from build123d import *

# Parameters (mm, degrees)
BOSS_EXTRUDE1_DEPTH = 30
SKETCH2_W           = 2.5
SKETCH2_H           = 5
CUT_EXTRUDE1_DEPTH  = 5
SKETCH3_R           = 8.1
CUT_EXTRUDE2_DEPTH  = 71
BOSS_EXTRUDE5_DEPTH = 4
CUT_EXTRUDE3_DEPTH  = 2
FILLET1_R           = 2


with BuildPart() as part:
    # Sketch1 → Boss-Extrude1 (new body)
    with BuildSketch(Plane(origin=(0, 0, 0), x_dir=(1, 0, 0), z_dir=(0, 1, 0))):
        with BuildLine():
            Line((8, -65), (8, 0))
            Line((8, 0), (58, 0))
            Line((58, 0), (58, -6.5))
            Line((58, -6.5), (55, -6.5))
            ThreePointArc((55, -6.5), (54.292893219, -6.792893219), (54, -7.5))
            Line((54, -7.5), (54, -9))
            ThreePointArc((54, -9), (54.292893219, -9.707106781), (55, -10))
            Line((55, -10), (60, -10))
            ThreePointArc((60, -10), (61.414213562, -9.414213562), (62, -8))
            Line((62, -8), (62, 0))
            Line((62, 0), (116, 0))
            Line((116, 0), (116, 5))
            Line((116, 5), (0, 5))
            Line((0, 5), (0, -10))
            Line((0, -10), (5, -10))
            Line((5, -10), (5, -57.5))
            Line((5, -57.5), (0, -57.5))
            Line((0, -57.5), (0, -63))
            ThreePointArc((0, -63), (0.585786438, -64.414213562), (2, -65))
            Line((2, -65), (8, -65))
        make_face()
    extrude(amount=BOSS_EXTRUDE1_DEPTH)

    # Sketch2 → Cut-Extrude1 (cut)
    with BuildSketch(Plane.ZY):
        with Locations((8.75, 15)):
            Rectangle(SKETCH2_W, SKETCH2_H)
        with Locations((58.75, 15)):
            Rectangle(SKETCH2_W, SKETCH2_H)
    extrude(amount=-CUT_EXTRUDE1_DEPTH, mode=Mode.SUBTRACT)

    # Sketch3 → Cut-Extrude2 (cut, through all)
    with BuildSketch(Plane(origin=(0, 0, -5), x_dir=(-1, 0, 0), z_dir=(0, 0, -1))):
        with Locations((-103, 12)):
            Circle(SKETCH3_R)
        with Locations((-75.8, 12)):
            Circle(SKETCH3_R)
    extrude(amount=-CUT_EXTRUDE2_DEPTH, mode=Mode.SUBTRACT)

    # Sketch8 → Boss-Extrude5 (add)
    with BuildSketch(Plane(origin=(116, 0, 0), x_dir=(0, 0, -1), z_dir=(1, 0, 0))):
        with BuildLine():
            Line((-8, 36), (-9.664100589, 33.503849117))
            ThreePointArc((-9.664100589, 33.503849117), (-9.914184053, 32.974017022), (-10, 32.394448725))
            Line((-10, 32.394448725), (-10, 30.32455532))
            ThreePointArc((-10, 30.32455532), (-9.974174915, 30.004190834), (-9.897366596, 29.692099788))
            Line((-9.897366596, 29.692099788), (0, 0))
            Line((0, 0), (0, 30))
            Line((0, 30), (-6, 30))
            Line((-6, 30), (-6, 36))
            Line((-6, 36), (-8, 36))
        make_face()
        with BuildLine():
            Line((5, 30), (5, 34))
            ThreePointArc((5, 34), (4.414213562, 35.414213562), (3, 36))
            Line((3, 36), (0, 36))
            Line((0, 36), (0, 30))
            Line((0, 30), (5, 30))
        make_face()
    extrude(amount=-BOSS_EXTRUDE5_DEPTH)

    # Sketch10 → Cut-Extrude3 (cut)
    with BuildSketch(Plane(origin=(0, 0, -5), x_dir=(-1, 0, 0), z_dir=(0, 0, -1))):
        Polygon((-112, 30), (-113, 25), (-113, 1.5), (-65.8, 1.5), (-65.8, 26), (0, 26), (0, 30), align=None)
        with BuildLine():
            ThreePointArc((-93, 16), (-92.414213562, 17.414213562), (-91, 18))
            Line((-91, 18), (-87.8, 18))
            ThreePointArc((-87.8, 18), (-86.385786438, 17.414213562), (-85.8, 16))
            Line((-85.8, 16), (-85.8, 10))
            ThreePointArc((-85.8, 10), (-86.385786438, 8.585786438), (-87.8, 8))
            Line((-87.8, 8), (-91, 8))
            ThreePointArc((-91, 8), (-92.414213562, 8.585786438), (-93, 10))
            Line((-93, 10), (-93, 16))
        make_face(mode=Mode.SUBTRACT)
    extrude(amount=-CUT_EXTRUDE3_DEPTH, mode=Mode.SUBTRACT)

    # Fillet1
    fillet1_edges = [part.edges().sort_by_distance(p)[0] for p in [
        (0, 13, -5),
        (0, 28, -3),
    ]]
    fillet(fillet1_edges, radius=FILLET1_R)


solid = part.part
The listing builds one solid part. Answer for the finished solid, in the listing's coordinates (mm). A direction names the side the tool comes from. Coordinates: 2 decimals unless noted, no trailing zeros. Write each loop counter-clockwise with the first axis right and the second up, starting at its lowest first coordinate (ties: lowest second). Pieces come first, ordered by that corner, then holes. Notation, with made-up numbers: M 70.25,-11 L 79.25,-11 A25 cw 79.25,1 Z; hole C 41.5,64 d9. An arc over 180 degrees is marked long. Put each result on its own line as item: value. Start each with the question number.
1. A cutting plane is placed at C-C on y = 28. Write down the section's boundary in (x, z), then the cut area to 3 significant figures.
2. Flat-ended cylindrical pins translate along their axes: P1, Ø10, axis at y = 22.5, z = 58, coming from the -X side; P2, Ø8, axis at x = 29, y = 29, coming from the +Z side; P3, Ø13, axis at x = 103, y = 12, coming from the -Z side; P4, Ø10, axis at y = 13.5, z = 11.5, coming from the +X side. Find the tip coordinate at first contact, or state that the pin passes through.
3. Which of the six approach directions +Z, -Z, +X, -X, +Y, -Y give full straight-line access (tool end or side, diameter ignored) to faces 1 (the flat face through (31, 30, -2)), 2 (the flat face through (2, 12.5, 59)), 3 (the flat face through (3, 24, 57.5)), 4 (the flat face through (62, 15, 4)), 5 (the flat face through (114, 33, 6))?
4. A cutting plane is placed at A-A on z = 2. Write down the section's boundary in (x, y), then the cut area to 3 significant figures.
5. A cutting plane is placed at D-D on x = 18. Write down the section's boundary in (y, z).
6. For a pull along Z with two mould halves and no side action, classify faces 6 (the flat face through (2, 15, 60)), 7 (the flat face through (34, 13, -5)), 8 (the flat face through (114, 15, 5)), 9 (the flat face through (8, 15, 33)) as pulls with the +Z half, pulls with the -Z half, needs draft (parallel to the pull), parting line crosses it, or undercut.
7. A cutting plane is placed at B-B on x = 75.8. Write down the section's boundary in (y, z), then the cut area to 3 significant figures.
8. Consider line 1 (X direction, y = 12, z = 2.5); line 2 (Y direction, x = 103, z = -0.7); line 3 (Y direction, x = 61.5, z = 0). Determine where each line is inside the solid, lowest interval first. Write a range as from..to.
Resolved:
1. outline: M 0,-1 A2 ccw 2,-3 L 112.4,-3 L 112.4,-5 L 116,-5 L 116,9.33 L 112,9.33 L 112,0 L 62,0 L 62,8 A2 ccw 60,10 L 55,10 A1 ccw 54,9 L 54,7.5 A1 ccw 55,6.5 L 58,6.5 L 58,0 L 8,0 L 8,65 L 2,65 A2 ccw 0,63 L 0,57.5 L 5,57.5 L 5,10 L 0,10 Z
1. area: 726 mm2
2. P1: stops at x = 0
2. P2: stops at z = 0
2. P3: passes through
2. P4: stops at x = 62
3. face 1: +Z, -Z, -X, +Y
3. face 2: -X
3. face 3: -X, +Y, -Y
3. face 4: +Z, +Y, -Y
3. face 5: +X, -X, +Y
4. outline: M 0,0 L 8,0 L 8,30 L 0,30 Z; M 58,0 L 62,0 L 62,30 L 58,30 Z; M 112,6 L 116,6 L 116,30 L 112,30 Z
4. area: 456 mm2
5. outline: M 0,-5 L 26,-5 L 26,-3 L 30,-3 L 30,0 L 0,0 Z
6. face 6: undercut
6. face 7: pulls with the -Z half
6. face 8: pulls with the +Z half
6. face 9: needs draft
7. outline: M 0,-5 L 1.5,-5 L 1.5,-3 L 3.9,-3 L 3.9,0 L 0,0 Z; M 20.1,-3 L 30,-3 L 30,0 L 20.1,0 Z
7. area: 44.4 mm2
8. line 1: x = 0..8, 58..62, 112..116
8. line 2: y = 0..3.9, 20.1..30
8. line 3: y = 0..30
